```python
from build123d import *

# Parameters (mm, degrees)
BOSS_EXTRUDE1_DEPTH = 20
SKETCH2_W           = 60
SKETCH2_H           = 30
BOSS_EXTRUDE2_DEPTH = 28
SKETCH3_R           = 6
CUT_EXTRUDE1_DEPTH  = 28


with BuildPart() as part:
    # Sketch1 → Boss-Extrude1 (new body)
    with BuildSketch(Plane.XY):
        Polygon((0, 75), (0, 30), (44, 30), (44, 40), (32, 40), (32, 52), (20, 52), (20, 75), align=None)
    extrude(amount=BOSS_EXTRUDE1_DEPTH)

    # Sketch2 → Boss-Extrude2 (add)
    with BuildSketch(Plane(origin=(0, 0, 0), x_dir=(-1, 0, 0), z_dir=(0, 0, -1))):
        with Locations((-30, 15)):
            Rectangle(SKETCH2_W, SKETCH2_H)
    extrude(amount=-BOSS_EXTRUDE2_DEPTH)

    # Sketch3 → Cut-Extrude1 (cut)
    with BuildSketch(Plane.XY.offset(28)):
        with Locations((48, 16)):
            Circle(SKETCH3_R)
    extrude(amount=-CUT_EXTRUDE1_DEPTH, mode=Mode.SUBTRACT)


solid = part.part
```
Design review of the part built by this model. Coordinates are the model's own, in mm. A direction names the side the tool comes from. Give positions to 0.01 mm unless a question says otherwise; leave off trailing zeros. Order: outer loops, then holes, each group sorted by start corner. A loop starts at its lowest first (then second) coordinate and runs counter-clockwise, first axis right, second up. Notation, with made-up numbers: (74.25, 60) - (113.25, 60) arc R20 cw to (113.25, 69) - close; hole circle Ø2 at (72, 75.25). An arc over 180 degrees is marked (long way). Use a Markdown table: item, result. Add a question column.
(1) Add section B-B on y = 16. Give the boundary of the cut face in (x, z), then the cut area to 3 significant figures.
(2) Clearance check with flat-ended pins moving along their axes: P1, Ø3, axis at y = 66, z = 18, coming from the -X side; P2, Ø5, axis at y = 35.5, z = 11, coming from the +X side; P3, Ø6, axis at y = 48, z = 14.5, coming from the +X side; P4, Ø4, axis at x = 41.5, y = 43, coming from the -Z side. State where each tip first meets the part, or that it passes through.
(3) Mouldability with a two-part tool opening along X and no side actions: class faces 4 (the face through (42, 16, 14)), 5 (the face through (10, 75, 10)), 6 (the face through (0, 37, 11)), 7 (the face through (60, 15, 14)) as +X half, -X half, draft (parallel to the pull), parting line (faces both ways), or undercut.
(4) Add section D-D on x = 37. Give the boundary of the cut face in (y, z).
(5) Machinability: for faces 1 (the face through (17, 48, 20)), 2 (the face through (26, 52, 10)), 3 (the face through (30, 15, 28)), which of the approach directions +Z, -Z, +X, -X, +Y, -Y give a long, thin tool a straight path to every point of the face, cutting with its end or side? Answer none if there is none.
(6) Add section A-A on x = 48. Give the boundary of the cut face in (y, z), then the cut area to 3 significant figures.
(7) Wall thickness on probe 1 along Z at (x, y) = (15, 34.5); probe 2 along Y at (x, z) = (56, 18.5); probe 3 along Y at (x, z) = (48, 19.75): over which ranges is each line inside the solid? List them lowest first. Write a range as [from, to].
(8) Add section C-C on z = 4.5. Give the boundary of the cut face in (x, y).
Report:
| question | item | result |
|---|---|---|
| 1 | outline | (0, 0) - (42, 0) - (42, 28) - (0, 28) - close; (54, 0) - (60, 0) - (60, 28) - (54, 28) - close |
| 1 | area | 1,340 mm² |
| 2 | P1 | stops at x = 0 |
| 2 | P2 | stops at x = 44 |
| 2 | P3 | stops at x = 32 |
| 2 | P4 | passes through |
| 3 | face 4 | undercut |
| 3 | face 5 | draft |
| 3 | face 6 | -X half |
| 3 | face 7 | +X half |
| 4 | outline | (0, 0) - (40, 0) - (40, 20) - (30, 20) - (30, 28) - (0, 28) - close |
| 5 | face 1 | +Z, +X, -X, +Y |
| 5 | face 2 | +Z, -Z, +X, +Y |
| 5 | face 3 | +Z, +X, -X, +Y, -Y |
| 6 | outline | (0, 0) - (10, 0) - (10, 28) - (0, 28) - close; (22, 0) - (30, 0) - (30, 28) - (22, 28) - close |
| 6 | area | 504 mm² |
| 7 | probe 1 | z = [0, 20] |
| 7 | probe 2 | y = [0, 30] |
| 7 | probe 3 | y = [0, 10], [22, 30] |
| 8 | outline | (0, 0) - (60, 0) - (60, 30) - (44, 30) - (44, 40) - (32, 40) - (32, 52) - (20, 52) - (20, 75) - (0, 75) - close; hole circle Ø12 at (48, 16) |
